```python
from build123d import *

# Parameters (mm, degrees)
TOOTHEXTRUDECUTGEARBELT01_DEPTH = 5.749999914
PATTERNGEARBELT01_COUNT         = 15
BOREREVOLVESKETCH_W             = 13.91999979
BOREREVOLVESKETCH_H             = 4


with BuildPart() as part:
    # SketchRevolveGearBelt01 → GearBelt01 (revolve)
    with BuildSketch(Plane(origin=(0, 0, 0), x_dir=(0, 0, -1), z_dir=(1, 0, 0)), mode=Mode.PRIVATE) as gearbelt01_sk:
        Polygon((6.959999895, 0), (6.959999895, 9.524999857), (6.949999896, 9.524999857), (6.949999896, 11.786304982), (8.063312621, 14.474079664), (6.954657199, 14.933299776), (5.749999914, 12.024999819), (5.749999914, 11.525000827), (-5.749999914, 11.525000827), (-5.749999914, 12.024999819), (-6.954657199, 14.933299776), (-8.063312621, 14.474079664), (-6.949999896, 11.786304982), (-6.949999896, 9.524999857), (-6.959999895, 9.524999857), (-6.959999895, 0), align=None)
    revolve(gearbelt01_sk.sketch.rotate(Axis((0, 0, 0), (0, 0, -1)), 90), axis=Axis((0, 0, 0), (0, 0, -1)))

    # SketchToothGearBelt01 → ToothExtrudeCutGearBelt01 (cut, symmetric)
    with BuildSketch(Plane.XY):
        with BuildLine():
            Line((-1.346605253, 11.013778629), (-1.109802523, 10.505953538))
            ThreePointArc((-1.109802523, 10.505953538), (-0.962199254, 10.337644266), (-0.747279414, 10.275000846))
            Line((-0.747279414, 10.275000846), (0.747279414, 10.275000846))
            ThreePointArc((0.747279414, 10.275000846), (0.962199254, 10.337644266), (1.109802523, 10.505953538))
            Line((1.109802523, 10.505953538), (1.346605253, 11.013778629))
            ThreePointArc((1.346605253, 11.013778629), (1.613174654, 11.292327669), (1.994209948, 11.351157242))
            Line((1.994209948, 11.351157242), (0, 13.891157204))
            Line((0, 13.891157204), (-1.994209948, 11.351157242))
            ThreePointArc((-1.994209948, 11.351157242), (-1.613174654, 11.292327669), (-1.346605253, 11.013778629))
        make_face()
    toothextrudecutgearbelt01 = extrude(amount=TOOTHEXTRUDECUTGEARBELT01_DEPTH, both=True, mode=Mode.SUBTRACT)

    # PatternGearBelt01: ToothExtrudeCutGearBelt01 ×15 about axis
    patterngearbelt01_axis = Axis((0, 0, 0), (0, 0, 1))
    for i in range(1, PATTERNGEARBELT01_COUNT):
        add(toothextrudecutgearbelt01.rotate(patterngearbelt01_axis, i * 360 / PATTERNGEARBELT01_COUNT), mode=Mode.SUBTRACT)

    # BoreRevolveSketch → BoreRevolveCut (revolve, cut)
    with BuildSketch(Plane(origin=(0, 0, 0), x_dir=(0, 0, -1), z_dir=(1, 0, 0)), mode=Mode.PRIVATE) as borerevolvecut_sk:
        with Locations((0, 2)):
            Rectangle(BOREREVOLVESKETCH_W, BOREREVOLVESKETCH_H)
    revolve(borerevolvecut_sk.sketch.rotate(Axis((0, 0, 0), (0, 0, -1)), 90), axis=Axis((0, 0, 0), (0, 0, -1)), mode=Mode.SUBTRACT)


solid = part.part
```
Can you work these out from the model? Positions are in its coordinate system, mm. A direction names the side the tool comes from. Coordinates: 2 decimals unless noted, no trailing zeros. Answer as a JSON object with one key per item and string values.
1) Thinking about a two-plate mould opening in Y: for faces 5 (the face through (-9.775, 3.165, 0.08)), 6 (the face through (0.006, -11.525, 0.08)), 7 (the face through (-2.402, 11.272, 0.08)), 8 (the face through (-2.64, 11.88, -5.81)), which applies, pulls with the +Y half, pulls with the -Y half, needs draft (parallel to the pull), parting line crosses it, or undercut?
Results:
{"face 5": "undercut", "face 6": "pulls with the -Y half", "face 7": "pulls with the +Y half", "face 8": "parting line crosses it"}
2) For faces 1 (the face through (4.17, 9.39, 0.08)), 2 (the face through (2.391, 11.274, 0.08)), 3 (the face through (6.048, -8.307, 0.08)), 4 (the face through (-10.22, -1.08, 0.08)), which set-ups out of +Z, -Z, +X, -X, +Y, -Y let a thin tool reach every point of the face, with its end or its side?
Results:
{"face 1": "+Y", "face 2": "+X, +Y", "face 3": "-Y", "face 4": "-X"}
3) If I drill on line 1 (Y direction, x = 0, z = 3.25) (3 decimals); line 2 (Z direction, x = 7, y = -6); line 3 (Z direction, x = 11, y = -4.75), over which ranges is the centre line in solid material (lowest first)?
Results:
{"line 1": "y = -11.525 to -4, 4 to 10.275", "line 2": "z = -6.96 to 6.96", "line 3": "z = -7.03 to -5.75, 5.75 to 7.03"}
4) For P1, Ø1.5, axis at y = 11, z = -2.5, coming from the +X side; P2, Ø3, axis at x = 11, z = -4, coming from the -Y side; P3, Ø5, axis at y = 3, z = -0.5, coming from the +X side, each with a flat end and sliding along its axis, tell me the tip position at first contact or that it passes through.
Results:
{"P1": "stops at x = 3.26", "P2": "stops at y = -4.34", "P3": "stops at x = 11.5"}
